Could you check a few things on this drawing? It's one solid part, dimensions in mm from its lowest x, y, z. Give positions to 0.01 mm unless a question says otherwise; leave off trailing zeros. Order: outer loops, then holes, each group sorted by start corner. A loop starts at its lowest first (then second) coordinate and runs counter-clockwise, first axis right, second up.
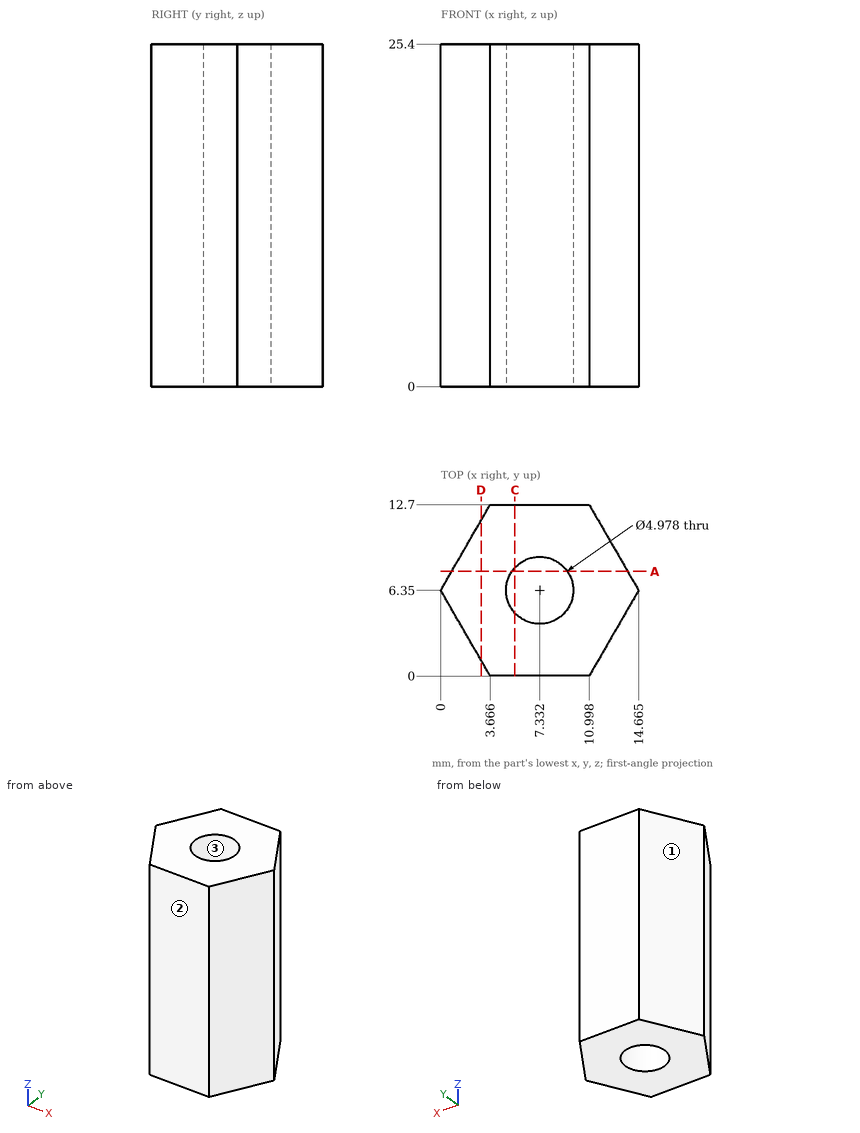
Q1. Thinking about a two-plate mould opening in X: for the marked faces 1, 2 and 3, which applies, released by +X, released by -X, zero draft, split by the parting line, or undercut?
Filled sheet:
face 1: released by -X
face 2: zero draft
face 3: undercut
Q2. If we section it at C-C on x = 5.5: List the corners of the cut face in (y, z) for me (1 decimal), plus the area to 3 significant figures.
Filled sheet:
outline: (0, 0) - (4.7, 0) - (4.7, 25.4) - (0, 25.4) - close; (8, 0) - (12.7, 0) - (12.7, 25.4) - (8, 25.4) - close
area: 237 mm2
Q3. I'm going to push a flat-ended pin straight in: P1, Ø3, axis at y = 9.5, z = 12, coming from the -X side. Where does the tip first touch, or does it pass through?
Filled sheet:
P1: stops at x = 0.95
Q4. I need wall thicknesses on L1, parallel to Y at x = 7.25, z = 9.75; L2, parallel to Y at x = 6.5, z = 14.5 (1 decimal); L3, parallel to Y at x = 3.5, z = 7 (1 decimal). Which ranges of each line are inside material? Lowest first, please.
Filled sheet:
L1: y = 0 to 3.86, 8.84 to 12.7
L2: y = 0 to 4, 8.7 to 12.7
L3: y = 0.3 to 12.4
Q5. If we section it at D-D on x = 3: List the corners of the cut face in (y, z) for me.
Filled sheet:
outline: (1.15, 0) - (11.55, 0) - (11.55, 25.4) - (1.15, 25.4) - close
Q6. If we section it at A-A on y = 7.75: List the corners of the cut face in (x, z) for me (1 decimal).
Filled sheet:
outline: (0.8, 0) - (5.3, 0) - (5.3, 25.4) - (0.8, 25.4) - close; (9.4, 0) - (13.9, 0) - (13.9, 25.4) - (9.4, 25.4) - close
